Here's the drawing with two shaded views (mm, measured from the low corner). I have some questions. Coordinates: 2 decimals unless noted, no trailing zeros. Loops run counter-clockwise (first coordinate to the right, second up) from the corner with the lowest first, then second, coordinate; pieces in that order, holes last.
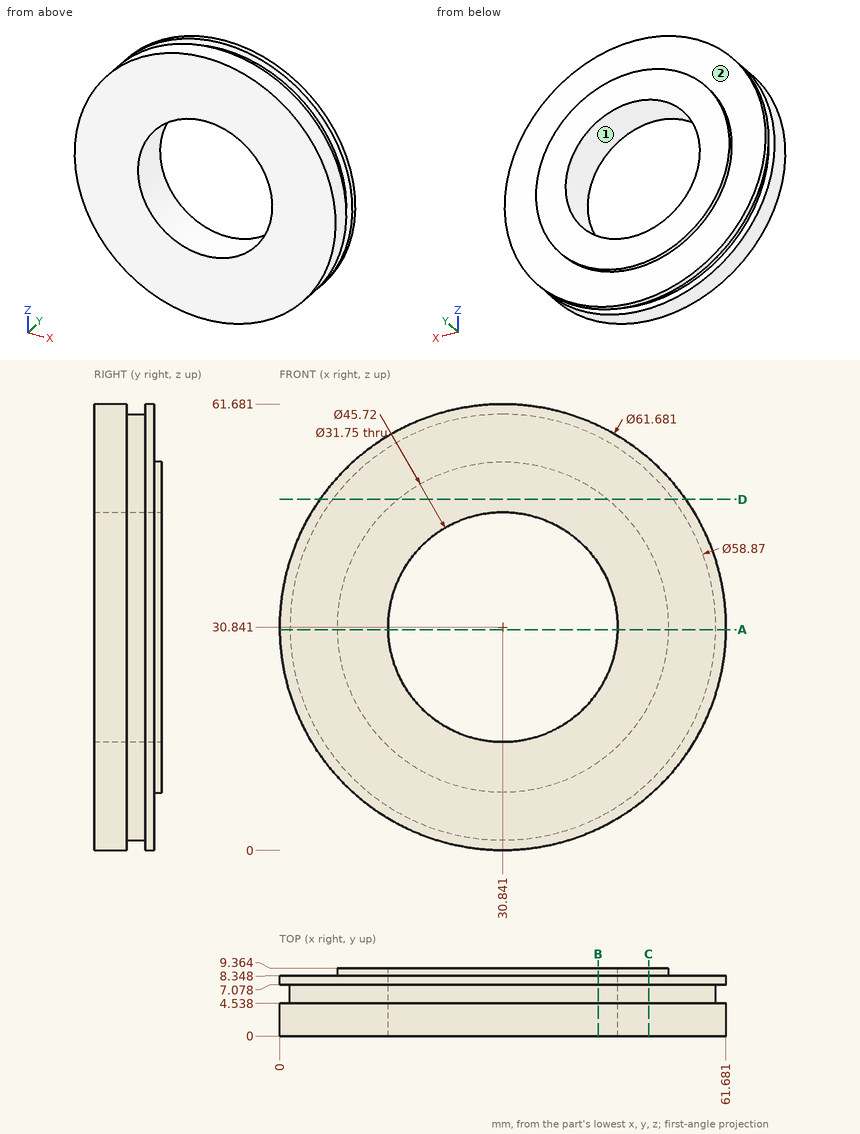
(1) I'm going to push a flat-ended pin straight in: pin 1 (4 mm diameter, centred on x = 49, y = 4.5, fed in from -Z). Where does the tip first touch, or does it pass through?
Check values:
pin 1: stops at z = 4.57
(2) I want a section at A-A on z = 30.5. Write out the boundary of the cut face in (x, y).
Check values:
outline: (0, 0) - (14.97, 0) - (14.97, 9.36) - (7.98, 9.36) - (7.98, 8.35) - (0, 8.35) - (0, 7.08) - (1.41, 7.08) - (1.41, 4.54) - (0, 4.54) - close; (46.71, 0) - (61.68, 0) - (61.68, 4.54) - (60.27, 4.54) - (60.27, 7.08) - (61.68, 7.08) - (61.68, 8.35) - (53.7, 8.35) - (53.7, 9.36) - (46.71, 9.36) - close
(3) If I drill on probe 1 along X at (y, z) = (6.25, 31.5); probe 2 along X at (y, z) = (0.5, 28.5); probe 3 along Z at (x, y) = (21, 7.25) (1 decimal), over which ranges is the centre line in solid material (lowest first)?
Check values:
probe 1: x = 1.41 to 14.98, 46.7 to 60.27
probe 2: x = 0.09 to 15.14, 46.54 to 61.59
probe 3: z = 1.6 to 18.4, 43.3 to 60.1
(4) I want a section at B-B on x = 44. Write out the boundary of the cut face in (y, z).
Check values:
outline: (0, 2.95) - (4.54, 2.95) - (4.54, 4.51) - (7.08, 4.51) - (7.08, 2.95) - (8.35, 2.95) - (8.35, 12.15) - (9.36, 12.15) - (9.36, 21.96) - (0, 21.96) - close; (0, 39.72) - (9.36, 39.72) - (9.36, 49.53) - (8.35, 49.53) - (8.35, 58.73) - (7.08, 58.73) - (7.08, 57.17) - (4.54, 57.17) - (4.54, 58.73) - (0, 58.73) - close
(5) If we mould it in two halves opening along Z, with no side actions, what happens to the marked faces 1 and 2? For each: released by +Z, released by -Z, zero draft, split by the parting line, or undercut.
Check values:
face 1: undercut
face 2: zero draft
(6) I want a section at C-C on x = 51. Write out the boundary of the cut face in (y, z), then the cut area to 3 significant figures.
Check values:
outline: (0, 7.5) - (4.54, 7.5) - (4.54, 9.39) - (7.08, 9.39) - (7.08, 7.5) - (8.35, 7.5) - (8.35, 20.06) - (9.36, 20.06) - (9.36, 41.62) - (8.35, 41.62) - (8.35, 54.18) - (7.08, 54.18) - (7.08, 52.29) - (4.54, 52.29) - (4.54, 54.18) - (0, 54.18) - close
area: 402 mm2
(7) I want a section at D-D on z = 48.5. Write out the boundary of the cut face in (x, y) (1 decimal).
Check values:
outline: (5.6, 0) - (56.1, 0) - (56.1, 4.5) - (54.4, 4.5) - (54.4, 7.1) - (56.1, 7.1) - (56.1, 8.3) - (45.4, 8.3) - (45.4, 9.4) - (16.3, 9.4) - (16.3, 8.3) - (5.6, 8.3) - (5.6, 7.1) - (7.3, 7.1) - (7.3, 4.5) - (5.6, 4.5) - close
